Check sheet for the drawn part. Datum: minimum x, y, z corner. Units: mm. Round coordinates to 2 decimals unless told otherwise and drop trailing zeros. Write each loop counter-clockwise with the first axis right and the second up, starting at its lowest first coordinate (ties: lowest second). Pieces come first, ordered by that corner, then holes.
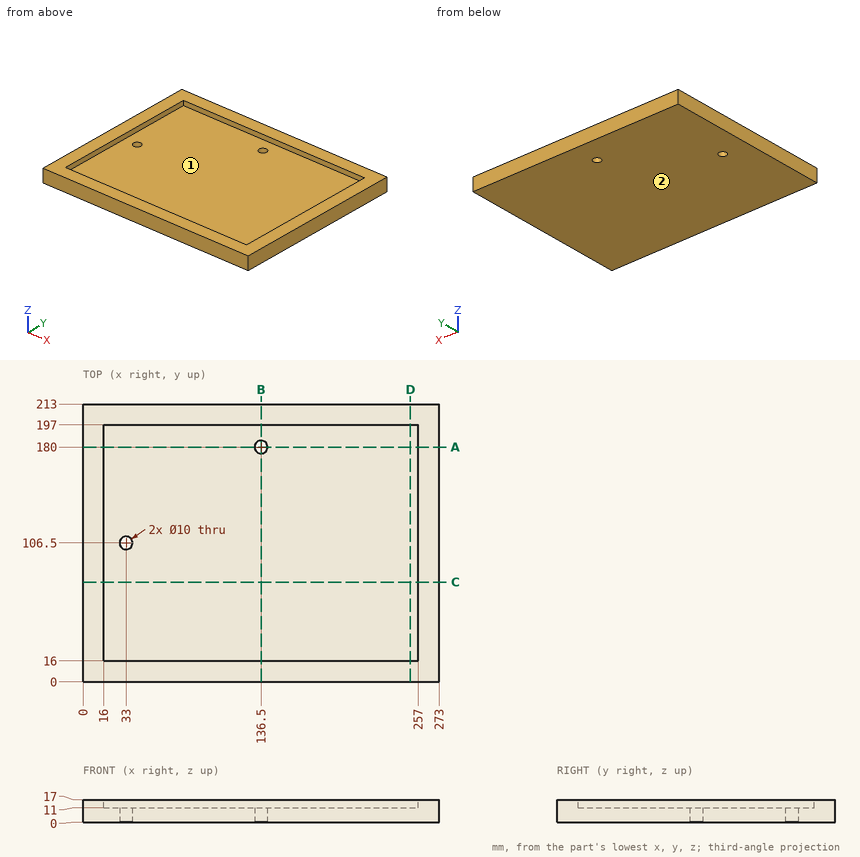
Q1. Sectioned sample at A-A (y = 180). Enter the section's corners in (x, z).
Recorded:
outline: (0, 0) - (131.5, 0) - (131.5, 11) - (16, 11) - (16, 17) - (0, 17) - close; (141.5, 0) - (273, 0) - (273, 17) - (257, 17) - (257, 11) - (141.5, 11) - close
Q2. Sectioned sample at D-D (x = 251). Enter the section's corners in (y, z), plus the area to 4 significant figures.
Recorded:
outline: (0, 0) - (213, 0) - (213, 17) - (197, 17) - (197, 11) - (16, 11) - (16, 17) - (0, 17) - close
area: 2,535 mm2
Q3. Sectioned sample at C-C (y = 76.5). Enter the section's corners in (x, z), plus the area to 4 significant figures.
Recorded:
outline: (0, 0) - (273, 0) - (273, 17) - (257, 17) - (257, 11) - (16, 11) - (16, 17) - (0, 17) - close
area: 3,195 mm2
Q4. Sectioned sample at B-B (x = 136.5). Enter the section's corners in (y, z), plus the area to 4 significant figures.
Recorded:
outline: (0, 0) - (175, 0) - (175, 11) - (16, 11) - (16, 17) - (0, 17) - close; (185, 0) - (213, 0) - (213, 17) - (197, 17) - (197, 11) - (185, 11) - close
area: 2,425 mm2
Q5. Material ranges on line 1 along X through (y, z) = (177, 14); line 2 along Y through (x, z) = (136.5, 7); line 3 along Y through (x, z) = (102, 11.5), recorded low to high.
Recorded:
line 1: x = 0 to 16, 257 to 273
line 2: y = 0 to 175, 185 to 213
line 3: y = 0 to 16, 197 to 213
Q6. Depth check by flat-ended pin: P1, Ø11.5, axis at x = 136.5, y = 180, coming from the -Z side; P2, Ø8, axis at x = 68, y = 54, coming from the +Z side. Enter the tip coordinate at first touch or a pass-through.
Recorded:
P1: stops at z = 0
P2: stops at z = 11
Q7. Release check for a two-part mould opening along X. For the marked faces 1 and 2 record: released by +X, released by -X, zero draft, split by the parting line, or undercut.
Recorded:
face 1: undercut
face 2: zero draft
